Build history of the part. All positions in model axes, mm. Give positions to 0.01 mm unless a question says otherwise; leave off trailing zeros. Loops run counter-clockwise (first coordinate to the right, second up) from the corner with the lowest first, then second, coordinate; pieces in that order, holes last. Notation, with made-up numbers: M 76,22.5 L 106,22.5 A19 ccw 106,55.5 Z; hole C 82,16 d2. An arc over 180 degrees is marked long. Put each result on its own line as item: value.
```python
from build123d import *

# Parameters (mm, degrees)
EXTRUDE1_DEPTH             = 300
EXTRUDE2_REACH             = 302.104
SKETCH2_R                  = 1.75
SKETCH_R                   = 3
SKETCH_R_2                 = 1.75
EXTRUDE4_DEPTH             = 3.5
CHAMFER1_SIZE              = 0.2
LPATTERN1_COUNT            = 15
LPATTERN1_PITCH            = 20
CHAMFER1_OF_LPATTERN1_SIZE = 0.2


with BuildPart() as part:
    # Sketch1 → Extrude1 (new body)
    with BuildSketch(Plane.XY):
        with BuildLine():
            Line((-4.3, -3.25), (4.3, -3.25))
            Line((4.3, -3.25), (4.5, -3.05))
            Line((4.5, -3.05), (4.5, 0.455012563))
            ThreePointArc((4.5, 0.455012563), (3.924845827, 0.712323349), (3.617735397, 1.2625))
            Line((3.617735397, 1.2625), (3.15008224, 1.2625))
            Line((3.15008224, 1.2625), (3.15008224, 1.7625))
            Line((3.15008224, 1.7625), (3.65008224, 1.7625))
            ThreePointArc((3.65008224, 1.7625), (3.973877727, 2.229724887), (4.5, 2.444987437))
            Line((4.5, 2.444987437), (4.5, 3.05))
            Line((4.5, 3.05), (4.3, 3.25))
            Line((4.3, 3.25), (-4.3, 3.25))
            Line((-4.3, 3.25), (-4.5, 3.05))
            Line((-4.5, 3.05), (-4.5, 2.444987437))
            ThreePointArc((-4.5, 2.444987437), (-3.973877727, 2.229724887), (-3.65008224, 1.7625))
            Line((-3.65008224, 1.7625), (-3.15008224, 1.7625))
            Line((-3.15008224, 1.7625), (-3.15008224, 1.2625))
            Line((-3.15008224, 1.2625), (-3.617735397, 1.2625))
            ThreePointArc((-3.617735397, 1.2625), (-3.924845827, 0.712323349), (-4.5, 0.455012563))
            Line((-4.5, 0.455012563), (-4.5, -3.05))
            Line((-4.5, -3.05), (-4.3, -3.25))
        make_face()
    extrude(amount=EXTRUDE1_DEPTH)

    # Sketch2 → Extrude2 (cut, up to next)
    with BuildSketch(Plane(origin=(0, 3.25, 0), x_dir=(1, 0, 0), z_dir=(0, 1, 0)), mode=Mode.PRIVATE) as extrude2_sk1:
        with Locations(Location((0, -10, 0), (0, 0, 270))):
            Circle(SKETCH2_R)
    extrude2_tool1 = extrude(extrude2_sk1.sketch, amount=-EXTRUDE2_REACH, mode=Mode.PRIVATE) & part.part
    extrude2 = extrude2_tool1.solids().sort_by_distance((0, 3.25, 10))[0]
    add(extrude2, mode=Mode.SUBTRACT)

    # Sketch → Extrude4 (cut)
    with BuildSketch(Plane(origin=(0, 3.25, 0), x_dir=(1, 0, 0), z_dir=(0, 1, 0))):
        with Locations(Location((0, -10, 0), (0, 0, 270))):
            Circle(SKETCH_R)
        with Locations(Location((0, -10, 0), (0, 0, 270))):
            Circle(SKETCH_R_2, mode=Mode.SUBTRACT)
    extrude4 = extrude(amount=-EXTRUDE4_DEPTH, mode=Mode.SUBTRACT)

    # Chamfer1
    chamfer1_edges = [part.edges().sort_by_distance(p)[0] for p in [
        (0, -3.25, 8.25),
        (0, 3.25, 7),
    ]]
    chamfer(chamfer1_edges, length=CHAMFER1_SIZE)

    # LPattern1: Extrude2, Extrude4 ×15
    with Locations(*[(0, 0, i * LPATTERN1_PITCH) for i in range(1, LPATTERN1_COUNT)]):
        add(extrude2, mode=Mode.SUBTRACT)
        add(extrude4, mode=Mode.SUBTRACT)

    # Chamfer1 of LPattern1
    chamfer1_of_lpattern1_edges = [part.edges().sort_by_distance(p)[0] for p in [
        (0, -3.25, 28.25),
        (0, 3.25, 27),
        (0, -3.25, 48.25),
        (0, 3.25, 47),
        (0, -3.25, 68.25),
        (0, 3.25, 67),
        (0, -3.25, 88.25),
        (0, 3.25, 87),
        (0, -3.25, 108.25),
        (0, 3.25, 107),
        (0, -3.25, 128.25),
        (0, 3.25, 127),
        (0, -3.25, 148.25),
        (0, 3.25, 147),
        (0, -3.25, 168.25),
        (0, 3.25, 167),
        (0, -3.25, 188.25),
        (0, 3.25, 187),
        (0, -3.25, 208.25),
        (0, 3.25, 207),
        (0, -3.25, 228.25),
        (0, 3.25, 227),
        (0, -3.25, 248.25),
        (0, 3.25, 247),
        (0, -3.25, 268.25),
        (0, 3.25, 267),
        (0, -3.25, 288.25),
        (0, 3.25, 287),
    ]]
    chamfer(chamfer1_of_lpattern1_edges, length=CHAMFER1_OF_LPATTERN1_SIZE)


solid = part.part
```
Q1. Slice it at B-B (z = 78). List the corners of the cut face in (x, y).
Here are the results:
outline: M -4.5,-3.05 L -4.3,-3.25 L 4.3,-3.25 L 4.5,-3.05 L 4.5,0.46 A1 cw 3.62,1.26 L 3.15,1.26 L 3.15,1.76 L 3.65,1.76 A1 cw 4.5,2.44 L 4.5,3.05 L 4.3,3.25 L -4.3,3.25 L -4.5,3.05 L -4.5,2.44 A1 cw -3.65,1.76 L -3.15,1.76 L -3.15,1.26 L -3.62,1.26 A1 cw -4.5,0.46 Z
Q2. Probe line 1 (X direction, y = -2.25, z = 70); line 2 (X direction, y = 1, z = 130); line 3 (X direction, y = 1.5, z = 161). List the from-to ranges inside material, lowest first. Write a range as from..to.
Here are the results:
line 1: -4.5..-1.75, 1.75..4.5
line 2: -3.71..-3, 3..3.71
line 3: -3.15..3.15
Q3. Drop a flat-ended pin along its axis: pin 1 Ø3 at (x, z) = (-1, 30) entering from +Y. Give the stop position or say it passes through.
Here are the results:
pin 1: y = -0.25
Q4. Mould opens along Z. For faces 1 (the flat face through (0, -0.25, 252)), 2 (the flat face through (0, 0, 300)), 3 (the flat face through (0, 0, 0)) say: pulls with the +Z half, pulls with the -Z half, needs draft (parallel to the pull), parting line crosses it, or undercut.
Here are the results:
face 1: undercut
face 2: pulls with the +Z half
face 3: pulls with the -Z half
Q5. Slice it at A-A (y = -1.5). State how many separate pieces and enclosed holes the cut face has, and give its area (3 significant figures).
Here are the results:
separate pieces: 1
enclosed holes: 15
area: 2,560 mm²
